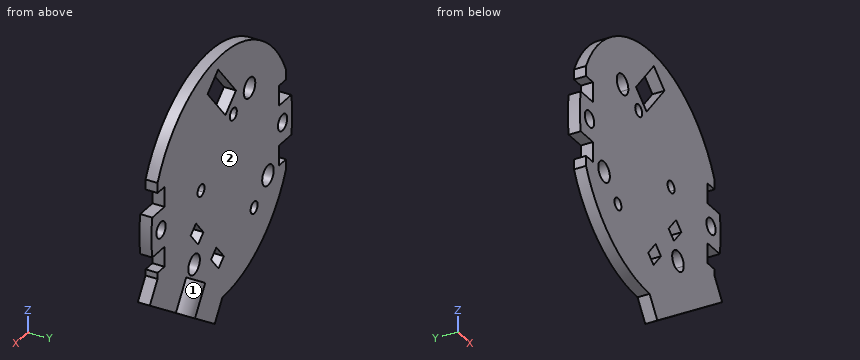
```python
from build123d import *

# Parameters (mm, degrees)
CROQUIS1_R              = 30.5
SALIENTE_EXTRUIR1_DEPTH = 3
CORTAR_EXTRUIR3_START   = -4
CORTAR_EXTRUIR3_DEPTH   = 4
CORTAR_EXTRUIR5_DEPTH   = 4
CROQUIS8_R              = 1.5
CORTAR_EXTRUIR6_DEPTH   = 10
CORTAR_EXTRUIR8_START   = -3
CROQUIS10_R             = 2
CORTAR_EXTRUIR8_DEPTH   = 3
CROQUIS11_R             = 2.5
CORTAR_EXTRUIR9_DEPTH   = 3
CROQUIS13_W             = 33.894616986
CROQUIS13_H             = 3
SALIENTE_EXTRUIR2_DEPTH = 6
CROQUIS14_R             = 3
SALIENTE_EXTRUIR3_DEPTH = 8
CROQUIS17_R             = 1.5
CORTAR_EXTRUIR10_DEPTH  = 7


with BuildPart() as part:
    # Croquis1 → Saliente-Extruir1 (new body)
    with BuildSketch(Plane(origin=(0, 0, 0), x_dir=(1, 0, 0), z_dir=(0, 1, 0))):
        with Locations(Location((0, 0, 0), (0, 0, 270))):
            Circle(CROQUIS1_R)
    extrude(amount=SALIENTE_EXTRUIR1_DEPTH)

    # Croquis5 → Cortar-Extruir3 (cut)
    with BuildSketch(Plane(origin=(0, 3, 0), x_dir=(1, 0, 0), z_dir=(0, 1, 0)).offset(CORTAR_EXTRUIR3_START)):
        with BuildLine():
            Line((28.814059068, 5), (30.087372767, 5))
            ThreePointArc((30.087372767, 5), (29.556634924, 7.526973624), (28.814059068, 10))
            Line((28.814059068, 10), (24.814059068, 10))
            Line((24.814059068, 10), (24.814059068, 5))
            Line((24.814059068, 5), (28.814059068, 5))
        make_face()
        with BuildLine():
            Line((30.087372767, -5), (28.814059068, -5))
            Line((28.814059068, -5), (24.814059068, -5))
            Line((24.814059068, -5), (24.814059068, -10))
            Line((24.814059068, -10), (28.814059068, -10))
            ThreePointArc((28.814059068, -10), (29.556634924, -7.526973624), (30.087372767, -5))
        make_face()
        with BuildLine():
            Line((-24.814059068, 5), (-24.814059068, 10))
            Line((-24.814059068, 10), (-28.814059068, 10))
            ThreePointArc((-28.814059068, 10), (-29.556634924, 7.526973624), (-30.087372767, 5))
            Line((-30.087372767, 5), (-28.814059068, 5))
            Line((-28.814059068, 5), (-24.814059068, 5))
        make_face()
        with BuildLine():
            Line((-28.814059068, -10), (-24.814059068, -10))
            Line((-24.814059068, -10), (-24.814059068, -5))
            Line((-24.814059068, -5), (-28.814059068, -5))
            Line((-28.814059068, -5), (-30.087372767, -5))
            ThreePointArc((-30.087372767, -5), (-29.556634924, -7.526973624), (-28.814059068, -10))
        make_face()
    extrude(amount=CORTAR_EXTRUIR3_DEPTH, mode=Mode.SUBTRACT)

    # Croquis7 → Cortar-Extruir5 (cut)
    with BuildSketch(Plane(origin=(0, 3, 0), x_dir=(1, 0, 0), z_dir=(0, 1, 0))):
        Polygon((1.428390211, 22.411430151), (-0.869743118, 20.483067322), (2.34419493, 16.652845106), (4.642328259, 18.581207935), align=None)
        Polygon((10.266719844, 11.878319058), (7.968586515, 9.949956229), (9.575555539, 8.034845121), (11.182524563, 6.119734013), (13.480657893, 8.048096842), align=None)
    extrude(amount=-CORTAR_EXTRUIR5_DEPTH, mode=Mode.SUBTRACT)

    # Croquis8 → Cortar-Extruir6 (cut)
    with BuildSketch(Plane(origin=(0, 3, 0), x_dir=(1, 0, 0), z_dir=(0, 1, 0))):
        Polygon((-6.154858987, -18.33209617), (1.558592329, -27.524629488), (6.154858987, -23.66790383), (-1.558592329, -14.475370512), align=None)
        with BuildLine():
            ThreePointArc((-9.5, -16), (-10.232233047, -14.232233047), (-12, -13.5))
            ThreePointArc((-12, -13.5), (-13.767766953, -17.767766953), (-9.5, -16))
        make_face()
        with BuildLine():
            ThreePointArc((14.5, 16), (10.232233047, 17.767766953), (12, 13.5))
            ThreePointArc((12, 13.5), (13.767766953, 14.232233047), (14.5, 16))
        make_face()
        with Locations(Location((-14, 15, 0), (0, 0, 270))):
            Circle(CROQUIS8_R)
        with BuildLine():
            Line((10.118033989, 0), (7.881966011, 0))
            ThreePointArc((7.881966011, 0), (8.464766865, -2.401258538), (10.5, -1))
            ThreePointArc((10.5, -1), (10.401258538, -0.464766865), (10.118033989, 0))
        make_face()
        with BuildLine():
            ThreePointArc((10.118033989, 0), (9, 0.5), (7.881966011, 0))
            Line((7.881966011, 0), (10.118033989, 0))
        make_face()
        with Locations(Location((-5, -13, 0), (0, 0, 270))):
            Circle(CROQUIS8_R)
    extrude(amount=-CORTAR_EXTRUIR6_DEPTH, mode=Mode.SUBTRACT)

    # Croquis10 → Cortar-Extruir8 (cut)
    with BuildSketch(Plane(origin=(0, 3, 0), x_dir=(1, 0, 0), z_dir=(0, 1, 0)).offset(CORTAR_EXTRUIR8_START)):
        with BuildLine():
            Line((-27.814059068, -12.515115586), (-27.814059068, -10))
            Line((-27.814059068, -10), (-28.814059068, -10))
            ThreePointArc((-28.814059068, -10), (-28.341972277, -11.268655974), (-27.814059068, -12.515115586))
        make_face()
        with BuildLine():
            Line((-28.814059068, 10), (-27.814059068, 10))
            Line((-27.814059068, 10), (-27.814059068, 12.515115586))
            ThreePointArc((-27.814059068, 12.515115586), (-28.341972277, 11.268655974), (-28.814059068, 10))
        make_face()
        with BuildLine():
            Line((27.814059069, -10), (27.814059069, -12.515115586))
            ThreePointArc((27.814059069, -12.515115586), (28.341972277, -11.268655974), (28.814059068, -10))
            Line((28.814059068, -10), (27.814059069, -10))
        make_face()
        with BuildLine():
            ThreePointArc((28.814059069, 10), (28.341972277, 11.268655974), (27.814059069, 12.515115586))
            Line((27.814059069, 12.515115586), (27.814059069, 10))
            Line((27.814059069, 10), (28.814059069, 10))
        make_face()
        with Locations(Location((-26.314059068, 0, 0), (0, 0, 270))):
            Circle(CROQUIS10_R)
        with Locations(Location((26.314059069, 0, 0), (0, 0, 270))):
            Circle(CROQUIS10_R)
    extrude(amount=CORTAR_EXTRUIR8_DEPTH, mode=Mode.SUBTRACT)

    # Croquis11 → Cortar-Extruir9 (cut)
    with BuildSketch(Plane(origin=(0, 3, 0), x_dir=(1, 0, 0), z_dir=(0, 1, 0))):
        with BuildLine():
            Line((-1.702166058, 31.453976389), (29.801261699, 10.204646058))
            ThreePointArc((29.801261699, 10.204646058), (17.614576459, 26.114683535), (-1.702166058, 31.453976389))
        make_face()
        with Locations(Location((-20, 10, 0), (0, 0, 270))):
            Circle(CROQUIS11_R)
    extrude(amount=-CORTAR_EXTRUIR9_DEPTH, mode=Mode.SUBTRACT)

    # Croquis13 → Saliente-Extruir2 (add)
    with BuildSketch(Plane(origin=(14.04954782, 0, -20.829311224), x_dir=(-0.8290375725550413, 0, -0.5591929034707476), z_dir=(0.5591929034707475, 0, -0.8290375725550412))):
        with Locations((0.344307973, 1.5)):
            Rectangle(CROQUIS13_W, CROQUIS13_H)
    extrude(amount=SALIENTE_EXTRUIR2_DEPTH)

    # Croquis14 → Saliente-Extruir3 (add)
    with BuildSketch(Plane(origin=(17.404705241, 0, -25.803536659), x_dir=(-0.8290375725550413, 0, -0.5591929034707476), z_dir=(0.5591929034707476, 0, -0.8290375725550413))):
        with Locations((0.004307973, 3)):
            Circle(CROQUIS14_R)
    extrude(amount=-SALIENTE_EXTRUIR3_DEPTH)

    # Croquis17 → Cortar-Extruir10 (cut)
    with BuildSketch(Plane(origin=(17.404705241, 0, -25.803536659), x_dir=(-0.8290375725550413, 0, -0.5591929034707476), z_dir=(0.5591929034707476, 0, -0.8290375725550413))):
        with Locations((0.004307973, 3)):
            Circle(CROQUIS17_R)
    extrude(amount=-CORTAR_EXTRUIR10_DEPTH, mode=Mode.SUBTRACT)


solid = part.part
```
Geometry: final body of the model. Coordinates: model frame, mm. Face numbers are marked on the shaded views. Give positions to 0.01 mm unless a question says otherwise; leave off trailing zeros. Write each loop counter-clockwise with the first axis right and the second up, starting at its lowest first coordinate (ties: lowest second). Pieces come first, ordered by that corner, then holes.
1. Line query: probe 1 along X at (y, z) = (1.65, 16); probe 2 along X at (y, z) = (1.2, -16); probe 3 along Z at (x, y) = (0.5, 2.85). Output: solid intervals per line, ascending.
2. Draft query along Z for the marked faces 1 and 2. Return one class per face: released by +Z, released by -Z, zero draft, split by the parting line, or undercut.
3. Section query B-B, the plane z = -14.5. Return loops of the section in (x, y).
4. Section query A-A, the plane x = -5. Return loops of the section in (y, z), then the cut area to 3 significant figures.
5. Section query C-C, the plane z = -29. Return loops of the section in (x, y).
6. Pin query (flat end, axial travel): P1, Ø10, axis at x = -7.5, z = -18.5, coming from the +Y side; P2, Ø0.8, axis at y = 2, z = 11.5, coming from the +X side; P3, Ø2.5, axis at x = -14, z = -15, coming from the +Y side; P4, Ø1.3, axis at y = 2, z = 11, coming from the -X side. Return the tip coordinate at first contact, or that it passes through.
Computed:
1. probe 1: x = -25.97 to -14.5, -9.5 to -3.38, -0.28 to 25.97
1. probe 2: x = -25.97 to -15.12, -12.88 to 9.5, 14.5 to 30.82
1. probe 3: z = -31.66 to -21.63, -18.85 to 16.93, 26.26 to 30.5
2. face 1: split by the parting line
2. face 2: zero draft
3. outline: (-26.83, 0) - (-15.41, 0) - (-15.41, 3) - (-26.83, 3) - close; (-12.59, 0) - (10, 0) - (10, 3) - (-12.59, 3) - close; (14, 0) - (29.81, 0) - (29.81, 3) - (14, 3) - close
4. outline: (0, -30.09) - (3, -30.09) - (3, 11.5) - (0, 11.5) - close; (0, 14.5) - (3, 14.5) - (3, 17.36) - (0, 17.36) - close; (0, 19.71) - (3, 19.71) - (3, 30.09) - (0, 30.09) - close
4. area: 164 mm2
5. outline: (-9.45, 0) - (12.67, 0) - (12.67, 3) - (-9.45, 3) - close
6. P1: stops at y = 3
6. P2: stops at x = 27.81
6. P3: passes through
6. P4: stops at x = -27.81
